Here's how the part is built. I have some questions about the finished solid (model axes, mm). A direction names the side the tool comes from. Give positions to 0.01 mm unless a question says otherwise; leave off trailing zeros. Write each loop counter-clockwise with the first axis right and the second up, starting at its lowest first coordinate (ties: lowest second). Pieces come first, ordered by that corner, then holes. Notation, with made-up numbers: (-23, 2) -> (11, 2) arc R20 cw to (11, 30) -> close; hole circle Ø11 at (15, 89.25). An arc over 180 degrees is marked (long way). Use CSV: the item, a comma, the result in double quotes. Start each with the question number.
(1) Suppose I cut it at A-A on y = 8.25. List the corners of the cut face in (x, z) for me.
(2) I need wall thicknesses on L1, parallel to X at y = 8.25, z = 4.5; L2, parallel to X at y = 19, z = -1; L3, parallel to Z at x = 7.5, y = 21. Which ranges of each line are inside material? Lowest first, please. Write a range as [from, to].
(3) Suppose I cut it at C-C on x = 8.5. List the corners of the cut face in (y, z) for me.
(4) For pin 1 Ø5 at (x, z) = (-17, 5) entering from +Y; pin 2 Ø5 at (y, z) = (5.5, 2) entering from -X; pin 3 Ø1.7 at (y, z) = (-6, 2.5) entering from -X, each with a flat end and sliding along its axis, tell me the tip position at first contact or that it passes through.
(5) Which directions (+Z, -Z, +X, -X, +Y, -Y) give clear straight access to the entire face, cutting with the end or side of a thin tool? Please do faces 1 (the flat face through (6, 8, 0)), 2 (the flat face through (9.77, 20.5, 4.93)).
(6) Suppose I cut it at D-D on y = -5.5. List the corners of the cut face in (x, z) for me, plus the area to 3 significant figures.
(7) If we mould it in two halves opening along X, with no side actions, what happens to faces 3 (the flat face through (10.8, 8.54, -1.48)), 4 (the flat face through (13.718, 8, 5)), 5 (the flat face through (0, -8.25, 5))? For each: pulls with the +X half, pulls with the -X half, needs draft (parallel to the pull), parting line crosses it, or undercut.
(8) Suppose I cut it at B-B on z = 6.5. List the corners of the cut face in (x, y) for me, plus the area to 3 significant figures.
Autodesk Inventor part; units mm, degrees
ref_plane "YZ Plane" through (0, 0, 0) normal (1, 0, 0) x (0, 1, 0)
ref_plane "XZ Plane" through (0, 0, 0) normal (0, 1, 0) x (-1, 0, 0)
ref_plane "XY Plane" through (0, 0, 0) normal (0, 0, 1) x (1, 0, 0)
sketch "Sketch1" plane through (0, 0, 0) normal (0, 0, 1) x (1, 0, 0)
  arc A0 (-5.5118, -5.25) -> (-5.5118, 21.75) centre (-8.0118, 8.25) ccw
  circle A1 centre (-7.8118, 8.25) radius 10 construction
  circle A2 centre (-7.8118, 8.25) radius 12.15 construction
  line L0 (-5.5118, -8.25) -> (-5.5118, -5.25) construction
  line L1 (7.4882, -8.25) -> (-5.5118, -8.25) construction
  line L2 (11.0118, -4.7265) -> (7.4882, -8.25) construction
  line L3 (11.0118, -4.7265) -> (11.0118, 21.2265) construction
  line L4 (11.0118, 21.2265) -> (7.4882, 24.75) construction
  line L5 (7.4882, 24.75) -> (-5.5118, 24.75) construction
  line L6 (-5.5118, 24.75) -> (-5.5118, 21.75) construction
  arc A3 (-5.5118, -5.25) -> (-5.5118, 21.75) centre (-8.0118, 8.25) ccw construction
  circle A4 centre (-7.8118, 8.25) radius 12.25
  circle A5 centre (-7.8118, 8.25) radius 13.25
  line L7 (-5.5118, 21.2989) -> (-5.5118, 24.75)
  line L8 (-5.5118, 24.75) -> (5.7178, 24.75)
  line L9 (5.7178, 24.75) -> (5.7178, -8.25)
  line L10 (5.7178, 24.75) -> (38.7178, 24.75) construction
  line L11 (5.7178, -8.25) -> (-5.5118, -8.25)
  line L12 (-5.5118, -8.25) -> (-5.5118, -4.7989)
  line L13 (13.7178, 16.3622) -> (5.7178, 16.3622)
  line L14 (5.7178, 16.3622) -> (5.7178, 0.5675)
  line L15 (5.7178, 0.5675) -> (13.7178, 0.5675)
  line L16 (13.7178, 0.5675) -> (13.7178, 16.3622)
  line L17 (13.7178, 16.3622) -> (5.7178, 0.5675) construction
  line L18 (5.7178, 16.3622) -> (13.7178, 0.5675) construction
  line L19 (13.7178, 0.5675) -> (5.7178, -8.25)
  line L20 (13.7178, 16.3622) -> (5.7178, 24.75)
  point P0 (0, 0)
  point P1 (9.7178, 8.4649)
  dimension "d0" = 24.5
  dimension "d1" = 26.5
  dimension "d2" = 90
  dimension "d7" = 8
extrude "Extrusion1" add sketch "Sketch1" along normal blind 10
sketch "Sketch2" plane through (0, 0, 0) normal (0, 0, -1) x (-1, 0, 0)
  line L0 (-5.7178, -8.25) -> (-5.7178, 24.75)
  circle A0 centre (7.8118, 8.25) radius 12.25
  line L1 (5.5118, -8.25) -> (-5.7178, -8.25)
  line L2 (5.5118, -4.7989) -> (5.5118, -8.25)
  arc A1 (5.5118, -4.7989) -> (5.5118, 21.2989) centre (7.8118, 8.25) ccw
  line L3 (5.5118, 24.75) -> (5.5118, 21.2989)
  line L4 (-5.7178, 24.75) -> (5.5118, 24.75)
  circle A2 centre (7.8118, 8.25) radius 13.25
  line L5 (-13.7178, 16.3622) -> (-5.7178, 24.75)
  line L6 (-13.7178, 0.5675) -> (-13.7178, 16.3622)
  line L7 (-5.7178, -8.25) -> (-13.7178, 0.5675)
  line L8 (-13.7178, 16.3622) -> (-5.7178, 24.75)
  line L9 (-13.7178, 0.5675) -> (-13.7178, 16.3622)
  line L10 (-5.7178, -8.25) -> (-13.7178, 0.5675)
  line L11 (-11.0118, 21.2265) -> (-11.0118, -4.7265) construction
  line L12 (-10.6722, 19.5554) -> (-10.6722, -2.7892)
  line L13 (-5.7178, -8.25) -> (-13.7178, 0.5675)
  line L14 (-10.6722, 19.5554) -> (11.6724, 19.5554) construction
  point P0 (0, 0)
  dimension "d8" = 90
extrude "Extrusion2" add sketch "Sketch2" along normal blind 3 draft -5 contours L7 L6 L5 L12 | A2 A1
properties part number "cellSTORM_inverted_objectiveadapter"
Geometry says:
1,outline,"(-21.06, 0) -> (-20.8, -3) -> (-20.32, -3) -> (-20.06, 0) -> (-20.06, 10) -> (-21.06, 10) -> close; (4.44, 0) -> (4.7, -3) -> (5.18, -3) -> (5.44, 0) -> (10.67, 0) -> (10.93, -3) -> (13.46, -3) -> (13.72, 0) -> (13.72, 10) -> (4.44, 10) -> close"
2,L1,"[-21.06, -20.06], [4.44, 13.72]"
2,L2,"[-15.41, -13.87], [-1.76, -0.22], [10.76, 11.08]"
2,L3,"[0, 10]"
3,outline,"(-5.18, 0) -> (21.83, 0) -> (21.83, 10) -> (-5.18, 10) -> close"
4,pin 1,"y = 19.69"
4,pin 2,"x = -21.06"
4,pin 3,"x = -5.51"
5,face 1,"-Z"
5,face 2,"+Z, -Z, +X, +Y"
6,outline,"(-5.51, 0) -> (8.21, 0) -> (8.21, 10) -> (-5.51, 10) -> close"
6,area,"137 mm²"
7,face 3,"undercut"
7,face 4,"pulls with the +X half"
7,face 5,"needs draft"
8,outline,"(-5.51, -8.25) -> (5.72, -8.25) -> (13.72, 0.57) -> (13.72, 16.36) -> (5.72, 24.75) -> (-5.51, 24.75) -> (-5.51, 21.3) arc R13.25 ccw (long way) to (-5.51, -4.8) -> close; hole circle Ø24.5 at (-7.81, 8.25)"
8,area,"431 mm²"
